```python
from build123d import *

# Parameters (mm, degrees)
ESQUISSE1_R        = 1.5
BOSS_EXTRU_1_DEPTH = 5
ESQUISSE2_W        = 5
ESQUISSE2_H        = 10
BOSS_EXTRU_2_DEPTH = 5


with BuildPart() as part:
    # Esquisse1 → Boss.-Extru.1 (new body)
    with BuildSketch(Plane.XY):
        Polygon((0, 0), (32, 0), (32, -5), (37, -5), (37, 0), (37, 18), (12, 18), (12, 47), (0, 47), align=None)
        with Locations((6, 32)):
            Circle(ESQUISSE1_R, mode=Mode.SUBTRACT)
        with Locations((31, 12)):
            Circle(ESQUISSE1_R, mode=Mode.SUBTRACT)
    extrude(amount=BOSS_EXTRU_1_DEPTH)

    # Esquisse2 → Boss.-Extru.2 (add)
    # profile 1 of 2: a face of its own
    with BuildSketch(Plane(origin=(0, 0, 0), x_dir=(-1, 0, 0), z_dir=(0, 0, -1))):
        with BuildLine():
            Line((-65, 0), (-37, 0))
            Line((-37, 0), (-37, 18))
            add(Edge.make_bspline(
                [(-75.5, 0), (-75.5, 5.982232529), (-67.685409636, 18), (-37, 18)],
                knots=[0, 0, 0, 0, 1, 1, 1, 1], degree=3))
            Line((-75.5, 0), (-70, 0))
            Line((-70, 0), (-70, -5))
            Line((-70, -5), (-65, -5))
            Line((-65, -5), (-65, 0))
        make_face()
    # profile 2 of 2: a face of its own
    with BuildSketch(Plane(origin=(0, 0, 0), x_dir=(-1, 0, 0), z_dir=(0, 0, -1))):
        Polygon((0, 60), (0, 0), (32, 0), (32, 75), (20, 75), (20, 60), align=None)
        with Locations((24.5, 10)):
            Rectangle(ESQUISSE2_W, ESQUISSE2_H, mode=Mode.SUBTRACT)
        with Locations((24.5, 30)):
            Rectangle(ESQUISSE2_W, ESQUISSE2_H, mode=Mode.SUBTRACT)
    extrude(amount=-BOSS_EXTRU_2_DEPTH)


solid = part.part
```
The listing builds one solid part. Answer for the finished solid, in the listing's coordinates (mm). A direction names the side the tool comes from. Coordinates: 2 decimals unless noted, no trailing zeros. Write each loop counter-clockwise with the first axis right and the second up, starting at its lowest first coordinate (ties: lowest second). Pieces come first, ordered by that corner, then holes. Notation, with made-up numbers: M 45.5,-22 L 73.5,-22 A22 cw 73.5,4 Z; hole C -29.5,-7 d8. An arc over 180 degrees is marked long. Use a Markdown table: item, result. Add a question column.
1. Section B-B (y = 32) is taken. Give the vertices of the cut face in (x, z).
2. Section A-A (x = 6) is taken. Give the vertices of the cut face in (y, z), plus the area to 3 significant figures.
3. Section C-C (z = 2) is taken. Count the separate pieces of the cut face and the enclosed holes in it, plus the area to 3 significant figures.
4. Straight lines are drawn through the part: line 1 along Y through (x, z) = (-26, 1.6); line 2 along Y through (x, z) = (31, 3.85); line 3 along Y through (x, z) = (6, 4). For each, find the intervals that lie inside material, in ascending order. Write a range as [from, to].
5. Which of the six approach directions +Z, -Z, +X, -X, +Y, -Y give full straight-line access (tool end or side, diameter ignored) to faces 1 (the flat face through (-27, 30, 2)), 2 (the flat face through (65, -3, 2)), 3 (the flat face through (12, 32, 2))?
6. For a pull along X with two mould halves and no side action, classify faces 4 (the flat face through (-22, 30, 2)), 5 (the flat face through (6, 47, 2)), 6 (the flat face through (0, 54, 2)), 7 (the flat face through (-32, 37, 2)) as +X half, -X half, draft (parallel to the pull), parting line (faces both ways), or undercut.
7. Given P1, Ø2.5, axis at x = 31, y = 12, coming from the -Z side; P2, Ø2.5, axis at x = -11, z = 2, coming from the +Y side; P3, Ø2.5, axis at x = 50, z = 3, coming from the -Y side; P4, Ø2.5, axis at y = -2.5, z = 2, coming from the -X side, each flat-ended and moving along its own axis, determine where each tip first touches the part or whether it passes through.
Data:
| question | item | result |
|---|---|---|
| 1 | outline | M -32,0 L -27,0 L -27,5 L -32,5 Z; M -22,0 L 4.5,0 L 4.5,5 L -22,5 Z; M 7.5,0 L 12,0 L 12,5 L 7.5,5 Z |
| 2 | outline | M 0,0 L 30.5,0 L 30.5,5 L 0,5 Z; M 33.5,0 L 47,0 L 47,5 L 33.5,5 Z |
| 2 | area | 220 mm2 |
| 3 | separate pieces | 1 |
| 3 | enclosed holes | 4 |
| 3 | area | 3,600 mm2 |
| 4 | line 1 | y = [0, 5], [15, 25], [35, 75] |
| 4 | line 2 | y = [0, 10.5], [13.5, 18] |
| 4 | line 3 | y = [0, 30.5], [33.5, 47] |
| 5 | face 1 | +Z, -Z |
| 5 | face 2 | +Z, -Z, -Y |
| 5 | face 3 | +Z, -Z, +X, +Y |
| 6 | face 4 | undercut |
| 6 | face 5 | draft |
| 6 | face 6 | +X half |
| 6 | face 7 | -X half |
| 7 | P1 | passes through |
| 7 | P2 | stops at y = 60 |
| 7 | P3 | stops at y = 0 |
| 7 | P4 | stops at x = 32 |
